from build123d import *

# Parameters (mm, degrees)
F1_W      = 50
F1_H      = 50
F2_DEPTH  = 1000
F3_W      = 20
F3_H      = 100
F4_DEPTH  = 900
F5_W      = 900
F5_H      = 90
F6_DEPTH  = 340
F7_W      = 860
F7_H      = 320
F8_DEPTH  = 70
F9_R      = 5
F10_DEPTH = 860


with BuildPart() as f2:
    # F1 (on Top) → F2 (new body)
    with BuildSketch(Plane.XY):
        with Locations((-25, -25)):
            Rectangle(F1_W, F1_H)
    extrude(amount=-F2_DEPTH)



with BuildPart() as f2b:
    # F1 (on Top) → F2, piece 2 (new body)
    with BuildSketch(Plane.XY):
        with Locations((-975, -25)):
            Rectangle(F1_W, F1_H)
    extrude(amount=-F2_DEPTH)


with BuildPart() as f2_1:
    add(f2.part)

    add(f2b.part)  # F4 merges F2b
    # F3 (on face) → F4 (join, through all)
    with BuildSketch(Plane.YZ.offset(-950)):
        with Locations((-20, -50)):
            Rectangle(F3_W, F3_H)
    extrude(amount=F4_DEPTH)

    # F5 (on face) → F6 (join)
    with BuildSketch(Plane.XZ.offset(30)):
        with Locations((-500, -45)):
            Rectangle(F5_W, F5_H)
    extrude(amount=F6_DEPTH)

    # F7 (on face) → F8 (cut)
    with BuildSketch(Plane.XY):
        with Locations((-500, -190)):
            Rectangle(F7_W, F7_H)
    extrude(amount=-F8_DEPTH, mode=Mode.SUBTRACT)

    # F9 (on face) → F10 (join, through all)
    with BuildSketch(Plane.YZ.offset(-930)):
        with Locations((-300, -5)):
            Circle(F9_R)
    extrude(amount=F10_DEPTH)


solid = f2_1.part
Work out the finished part from the listing and answer in its coordinate system (mm). A direction names the side the tool comes from. Coordinates: 2 decimals unless noted, no trailing zeros. Loops run counter-clockwise (first coordinate to the right, second up) from the corner with the lowest first, then second, coordinate; pieces in that order, holes last. Notation, with made-up numbers: M -13,-17 L 26,-17 A30 cw 26,12 Z; hole C 38,8 d4. An arc over 180 degrees is marked long. Answer in a Markdown table with one row per item. Add a question column.
1. The mould has two halves that part along Y. Classify faces 1 (the flat face through (-25, 0, -493)), 2 (the flat face through (-930, -192, -35)), 3 (the flat face through (-506, -188, -70)), 4 (the flat face through (-25, -25, -1000)): pulls with the +Y half, pulls with the -Y half, needs draft (parallel to the pull), parting line crosses it, or undercut.
2. Find section B-B, the plane x = -357. Write down the section's boundary in (y, z), then the cut area to 3 significant figures.
3. Flat-ended cylindrical pins translate along their axes: P1, Ø4, axis at x = -448, y = -89.5, coming from the -Z side; P2, Ø3, axis at x = -708.5, z = -94.5, coming from the -Y side; P3, Ø6, axis at x = -672, y = -18.5, coming from the -Z side. Find the tip coordinate at first contact, or state that the pin passes through.
4. A tool of negligible diameter and unlimited length cuts with its end or side. For faces 5 (the flat face through (-50, -208, -46)), 6 (the flat face through (-950, -208, -46)), 7 (the flat face through (-506, -350, -35)), from which of +Z, -Z, +X, -X, +Y, -Y can it reach the whole face along a straight path? Write none if from no direction.
5. Find section C-C, the plane y = -117.5. Write down the section's boundary in (x, z).
6. Find section A-A, the plane z = -580.5. Write down the section's boundary in (x, y), then the cut area to 3 significant figures.
7. Consider L1, parallel to Y at x = -84.5, z = -68; L2, parallel to Z at x = -219, y = -181; L3, parallel to Y at x = -61.5, z = -94. Determine where each line is inside the solid, lowest interval first.
Reported:
| question | item | result |
|---|---|---|
| 1 | face 1 | pulls with the +Y half |
| 1 | face 2 | undercut |
| 1 | face 3 | undercut |
| 1 | face 4 | needs draft |
| 2 | outline | M -370,-90 L -30,-90 L -30,-100 L -10,-100 L -10,0 L -30,0 L -30,-70 L -350,-70 L -350,0 L -370,0 Z; C -300,-5 d10 |
| 2 | area | 10,300 mm^2 |
| 3 | P1 | stops at z = -90 |
| 3 | P2 | stops at y = -30 |
| 3 | P3 | stops at z = -100 |
| 4 | face 5 | +Z, -Z, +X, -Y |
| 4 | face 6 | +Z, -Z, -X, -Y |
| 4 | face 7 | +Z |
| 5 | outline | M -950,-90 L -50,-90 L -50,0 L -70,0 L -70,-70 L -930,-70 L -930,0 L -950,0 Z |
| 6 | outline | M -1000,-50 L -950,-50 L -950,0 L -1000,0 Z; M -50,-50 L 0,-50 L 0,0 L -50,0 Z |
| 6 | area | 5,000 mm^2 |
| 7 | L1 | y = -370 to -350, -30 to -10 |
| 7 | L2 | z = -90 to -70 |
| 7 | L3 | y = -30 to -10 |
